from build123d import *

# Parameters (mm, degrees)
BOSS_EXTRUDE1_DEPTH = 127


with BuildPart() as part:
    # Sketch2 → Boss-Extrude1 (new body, symmetric)
    with BuildSketch(Plane.XY):
        with BuildLine():
            Line((0, 0), (0, 50.8))
            Line((0, 50.8), (6.35, 50.8))
            Line((6.35, 50.8), (6.35, 12.7))
            ThreePointArc((6.35, 12.7), (8.209871939, 8.209871939), (12.7, 6.35))
            Line((12.7, 6.35), (50.8, 6.35))
            Line((50.8, 6.35), (50.8, 0))
            Line((50.8, 0), (0, 0))
        make_face()
    extrude(amount=BOSS_EXTRUDE1_DEPTH, both=True)


solid = part.part
Geometry check sheet. Reference: the model listing, model coordinates, mm. A direction names the side the tool comes from. Round coordinates to 2 decimals unless told otherwise and drop trailing zeros. Loops run counter-clockwise (first coordinate to the right, second up) from the corner with the lowest first, then second, coordinate; pieces in that order, holes last. Notation, with made-up numbers: (85.5, 49) -> (140.5, 49) arc R23 cw to (140.5, 68) -> close; hole circle Ø11 at (89.25, 64.5). An arc over 180 degrees is marked (long way). Answer as a JSON object with one key per item and string values. Group by question number.
Item 1: Cross-section at A-A, the plane z = 2.5. Record the cut outline in (x, y), plus the area to 3 significant figures.
Item 2: Thickness scan on line 1 along Y through (x, z) = (36, 4.5); line 2 along Y through (x, z) = (8, -34). Record the ranges inside material, lowest first.
Item 3: Depth check by flat-ended pin: pin 1 Ø3 at (x, z) = (14, -70.5) entering from +Y; pin 2 Ø1 at (y, z) = (7.5, 27) entering from +X; pin 3 Ø11.5 at (x, z) = (33.5, 63) entering from +Y. Enter the tip coordinate at first touch or a pass-through.
Item 4: Cross-section at B-B, the plane y = 28.5. Record the cut outline in (x, z).
Item 5: Set-up check for faces 1 (the face through (6.35, 32, 2)), 2 (the face through (50.8, 3, 2)): record each of +Z, -Z, +X, -X, +Y, -Y from which the full face is reachable in a straight line by a thin tool's end or side.
Determined:
{
 "1": {"outline": "(0, 0) -> (50.8, 0) -> (50.8, 6.35) -> (12.7, 6.35) arc R6.35 cw to (6.35, 12.7) -> (6.35, 50.8) -> (0, 50.8) -> close", "area": "613 mm²"},
 "2": {"line 1": "y = 0 to 6.35", "line 2": "y = 0 to 8.43"},
 "3": {"pin 1": "stops at y = 6.35", "pin 2": "stops at x = 9.9", "pin 3": "stops at y = 6.35"},
 "4": {"outline": "(0, -127) -> (6.35, -127) -> (6.35, 127) -> (0, 127) -> close"},
 "5": {"face 1": "+Z, -Z, +X, +Y", "face 2": "+Z, -Z, +X, +Y, -Y"}
}
